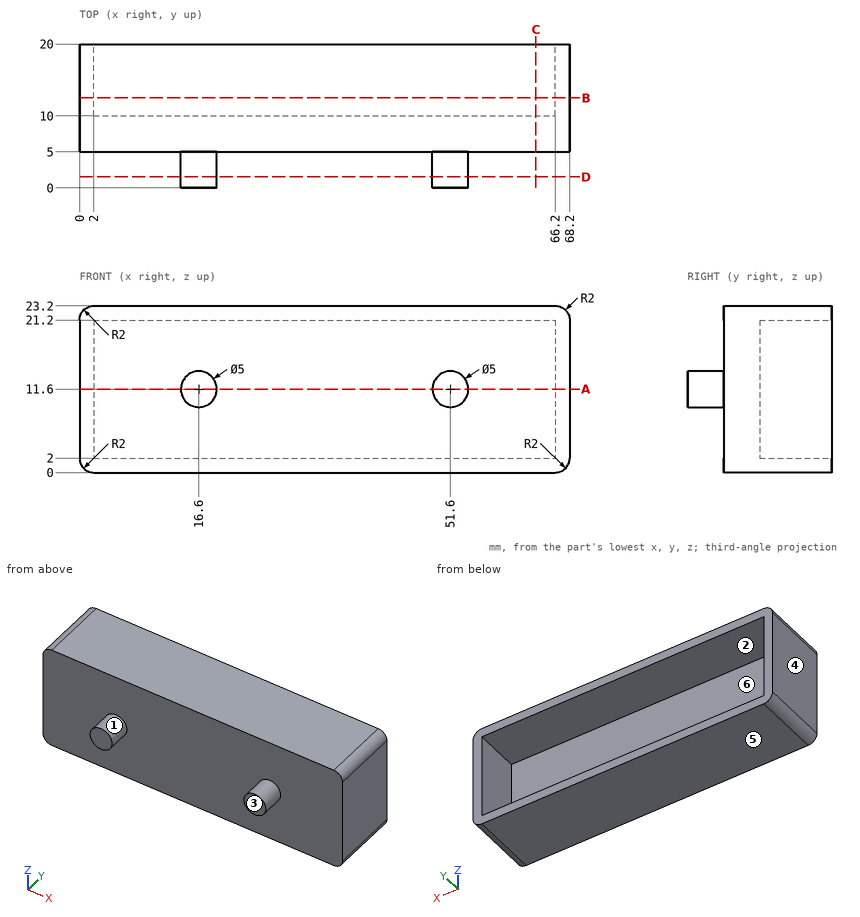
Answer from the drawing. Dimensions are ordinates in mm from the lowest x, y and z of the part. A direction names the side the tool comes from. Round coordinates to 2 decimals unless told otherwise and drop trailing zeros. Write each loop counter-clockwise with the first axis right and the second up, starting at its lowest first coordinate (ties: lowest second). Pieces come first, ordered by that corner, then holes. Notation, with made-up numbers: M 35.25,82.25 L 84.25,82.25 A22 cw 84.25,91.25 Z; hole C -10.75,-2 d8. An arc over 180 degrees is marked long. Write each question's results on one line, items separated by ' | '. Start each with the question number.
Item 1: The mould has two halves that part along Z. Classify the marked faces 4, 5 and 6: +Z half, -Z half, draft (parallel to the pull), parting line (faces both ways), or undercut.
Item 2: Find section C-C on x = 63.5. Write down the section's boundary in (y, z), and give its area (3 significant figures).
Item 3: Given pin 1 Ø6 at (x, z) = (38, 9.5) entering from +Y; pin 2 Ø11.5 at (x, z) = (37.5, 9.5) entering from -Y, each flat-ended and moving along its own axis, determine where each tip first touches the part or whether it passes through.
Item 4: Find section A-A on z = 11.6. Write down the section's boundary in (x, y).
Item 5: Straight lines are drawn through the part: probe 1 along Z at (x, y) = (7.5, 11); probe 2 along X at (y, z) = (11, 6.25); probe 3 along X at (y, z) = (2.5, 11.75). For each, find the intervals that lie inside material, in ascending order.
Item 6: Find section D-D on y = 1.5. Write down the section's boundary in (x, z), and give its area (3 significant figures).
Item 7: Which of the six approach directions +Z, -Z, +X, -X, +Y, -Y give full straight-line access (tool end or side, diameter ignored) to the marked faces 1, 2 and 3?
Item 8: Find section B-B on y = 12.5. Write down the section's boundary in (x, z), and give its area (3 significant figures).
Answer block:
1) face 4: draft | face 5: -Z half | face 6: undercut
2) outline: M 5,0 L 20,0 L 20,2 L 10,2 L 10,21.2 L 20,21.2 L 20,23.2 L 5,23.2 Z | area: 156 mm²
3) pin 1: stops at y = 10 | pin 2: stops at y = 5
4) outline: M 0,5 L 14.1,5 L 14.1,0 L 19.1,0 L 19.1,5 L 49.1,5 L 49.1,0 L 54.1,0 L 54.1,5 L 68.2,5 L 68.2,20 L 66.2,20 L 66.2,10 L 2,10 L 2,20 L 0,20 Z
5) probe 1: z = 0 to 2, 21.2 to 23.2 | probe 2: x = 0 to 2, 66.2 to 68.2 | probe 3: x = 14.1 to 19.1, 49.1 to 54.1
6) outline: C 16.6,11.6 d5; C 51.6,11.6 d5 | area: 39.3 mm²
7) face 1: -Y | face 2: +Y | face 3: +Z, -Z, +X, -X, -Y
8) outline: M 0,2 A2 ccw 2,0 L 66.2,0 A2 ccw 68.2,2 L 68.2,21.2 A2 ccw 66.2,23.2 L 2,23.2 A2 ccw 0,21.2 Z; hole M 2,2 L 66.2,2 L 66.2,21.2 L 2,21.2 Z | area: 346 mm²
